Could you check a few things on this drawing? It's one solid part, dimensions in mm from its lowest x, y, z. Coordinates: 2 decimals unless noted, no trailing zeros. Write each loop counter-clockwise with the first axis right and the second up, starting at its lowest first coordinate (ties: lowest second). Pieces come first, ordered by that corner, then holes. Notation, with made-up numbers: (68.5, 30.25) - (112.5, 30.25) arc R16 ccw to (112.5, 56.25) - close; hole circle Ø3 at (78.25, 58.5). An arc over 180 degrees is marked (long way). Use one line per item in the form item = value. Start each with the question number.
(1) If we section it at D-D on z = 3.55: Please give me the cut outline in (x, y).
(2) If we section it at B-B on y = 5.65: Please give me the cut outline in (x, z), then the cut area to 4 significant figures.
(3) For pin 1 Ø4.5 at (x, y) = (52.3, 32.3) entering from -Z; pin 2 Ø3.5 at (x, y) = (5.65, 36.65) entering from +Z, each with a flat end and sliding along its axis, tell me the tip position at first contact or that it passes through.
(4) If I drill on probe 1 along X at (y, z) = (5.5, 4.5); probe 2 along Y at (x, z) = (5.65, 1.75); probe 3 along Y at (x, z) = (52.3, 2.1), over which ranges is the centre line in solid material (lowest first)? Write a range as from..to.
(5) Thinking about a two-plate mould opening in X: for the marked faces 1, 2 and 3, which applies, pulls with the +X half, pulls with the -X half, needs draft (parallel to the pull), parting line crosses it, or undercut?
(6) If we section it at A-A on x = 5.65: Please give me the cut outline in (y, z), then the cut area to 4 significant figures.
(7) If we section it at C-C on x = 21.15: Please give me the cut outline in (y, z), then the cut area to 3 significant figures.
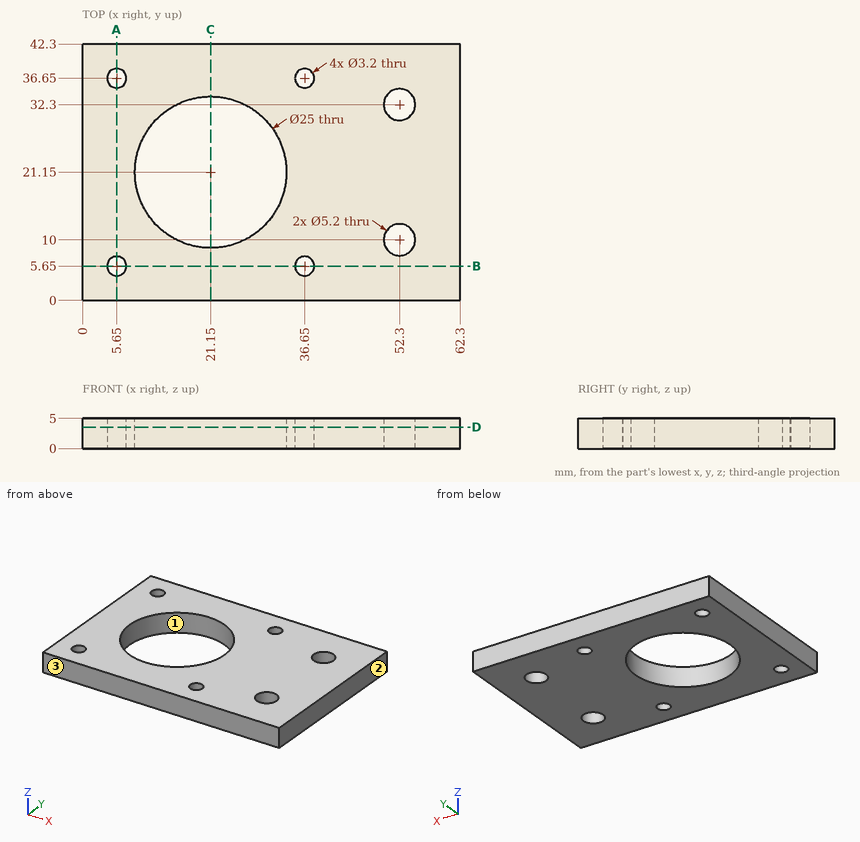
Reported:
q1.outline = (0, 0) - (62.3, 0) - (62.3, 42.3) - (0, 42.3) - close; hole circle Ø3.2 at (5.65, 5.65); hole circle Ø3.2 at (5.65, 36.65); hole circle Ø25 at (21.15, 21.15); hole circle Ø3.2 at (36.65, 5.65); hole circle Ø3.2 at (36.65, 36.65); hole circle Ø5.2 at (52.3, 10); hole circle Ø5.2 at (52.3, 32.3)
q2.outline = (0, 0) - (4.05, 0) - (4.05, 5) - (0, 5) - close; (7.25, 0) - (35.05, 0) - (35.05, 5) - (7.25, 5) - close; (38.25, 0) - (62.3, 0) - (62.3, 5) - (38.25, 5) - close
q2.area = 279.5 mm2
q3.pin_1 = through
q3.pin_2 = 5
q4.probe_1 = 0..4.06, 7.24..35.06, 38.24..62.3
q4.probe_2 = 0..4.05, 7.25..35.05, 38.25..42.3
q4.probe_3 = 0..7.4, 12.6..29.7, 34.9..42.3
q5.face_1 = undercut
q5.face_2 = pulls with the +X half
q5.face_3 = needs draft
q6.outline = (0, 0) - (4.05, 0) - (4.05, 5) - (0, 5) - close; (7.25, 0) - (35.05, 0) - (35.05, 5) - (7.25, 5) - close; (38.25, 0) - (42.3, 0) - (42.3, 5) - (38.25, 5) - close
q6.area = 179.5 mm2
q7.outline = (0, 0) - (8.65, 0) - (8.65, 5) - (0, 5) - close; (33.65, 0) - (42.3, 0) - (42.3, 5) - (33.65, 5) - close
q7.area = 86.5 mm2
